Can you work these out from the model? Positions are in its coordinate system, mm. Face numbers are marked on the shaded views. A direction names the side the tool comes from. Give positions to 0.01 mm unless a question says otherwise; leave off trailing zeros. Write each loop counter-clockwise with the first axis right and the second up, starting at its lowest first coordinate (ties: lowest second). Pieces come first, ordered by that corner, then holes.
1. On a 3-axis mill with a long thin cutter (end or side, diameter ignored), from which of +Z, -Z, +X, -X, +Y, -Y can I reach the whole of each face in a straight line? I mean the marked faces 1, 2, 3 and 4. Say none if no direction works.
2. Suppose I cut it at B-B (z = -6.5). Please give me the cut outline in (x, y), and give its area (3 significant figures).
3. Thinking about a two-plate mould opening in X: for the marked faces 5, 6, 7 and 8, which applies, pulls with the +X half, pulls with the -X half, needs draft (parallel to the pull), parting line crosses it, or undercut?
4. I'm going to push flat-ended pins straight in: pin 1 (3 mm diameter, centred on y = -4, z = -6, fed in from -X); pin 2 (3 mm diameter, centred on x = 11, y = -2, fed in from +Z); pin 3 (5 mm diameter, centred on x = 7, z = -4, fed in from +Y); pin 4 (4.5 mm diameter, centred on x = 11, z = 1.5, fed in from -Y). Where does each tip first touch, or does it pass through?
5. Suppose I cut it at D-D (z = 0). Please give me the cut outline in (x, y) (3 decimals), and give its area (3 significant figures).
6. If I drill on probe 1 along X at (y, z) = (1, -6.5); probe 2 along Z at (x, y) = (-10.35, 0.7); probe 3 along X at (y, z) = (8, 0) (3 decimals), over which ranges is the centre line in solid material (lowest first)?
7. Suppose I cut it at C-C (y = -6.5). Please give me the cut outline in (x, z).
8. Suppose I cut it at A-A (x = 10.35). Please give me the cut outline in (y, z).
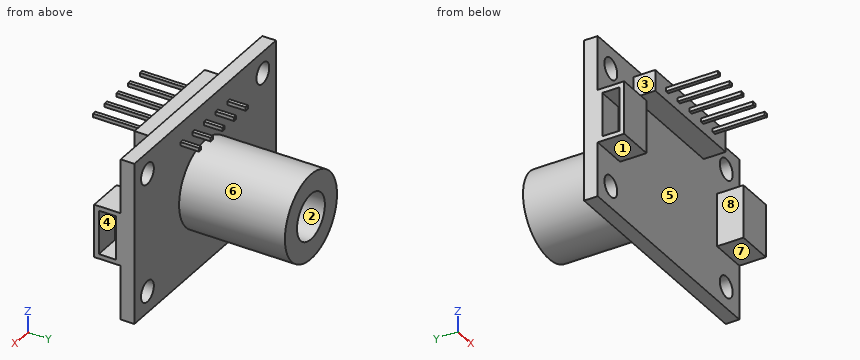
```python
from build123d import *

# Parameters (mm, degrees)
SKETCH1_W                = 25.4
SKETCH1_H                = 17.7
SKETCH1_R                = 1.15
BOSS_EXTRUDE1_DEPTH      = 1.5
SKETCH2_R                = 4.675
BOSS_EXTRUDE2_DEPTH      = 11.6
SKETCH3_R                = 2.5
CUT_EXTRUDE1_DEPTH       = 8
SKETCH4_W                = 4
SKETCH4_H                = 5.8
BOSS_EXTRUDE3_DEPTH      = 2.9
SKETCH5_W                = 4.8
SKETCH5_H                = 1.9
CUT_EXTRUDE2_DEPTH       = 2.9
SKETCH6_W                = 12.6
SKETCH6_H                = 2.3
BOSS_EXTRUDE4_DEPTH      = 2.4
SKETCH7_W                = 0.4
SKETCH7_H                = 0.4
BOSS_EXTRUDE5_DEPTH      = 5.7
BOSS_EXTRUDE5_DEPTH_BACK = 5.9


with BuildPart() as part:
    # Sketch1 → Boss-Extrude1 (new body)
    with BuildSketch(Plane(origin=(0, 0, 0), x_dir=(1, 0, 0), z_dir=(0, 1, 0))):
        Rectangle(SKETCH1_W, SKETCH1_H)
        with Locations((10.35, 6.5)):
            Circle(SKETCH1_R, mode=Mode.SUBTRACT)
        with Locations((10.35, -6.5)):
            Circle(SKETCH1_R, mode=Mode.SUBTRACT)
        with Locations((-10.35, -6.5)):
            Circle(SKETCH1_R, mode=Mode.SUBTRACT)
        with Locations((-10.35, 6.5)):
            Circle(SKETCH1_R, mode=Mode.SUBTRACT)
    extrude(amount=BOSS_EXTRUDE1_DEPTH)

    # Sketch2 → Boss-Extrude2 (add)
    with BuildSketch(Plane(origin=(0, 1.5, 0), x_dir=(1, 0, 0), z_dir=(0, 1, 0))):
        Circle(SKETCH2_R)
    extrude(amount=BOSS_EXTRUDE2_DEPTH)

    # Sketch3 → Cut-Extrude1 (cut)
    with BuildSketch(Plane(origin=(0, 13.1, 0), x_dir=(1, 0, 0), z_dir=(0, 1, 0))):
        Circle(SKETCH3_R)
    extrude(amount=-CUT_EXTRUDE1_DEPTH, mode=Mode.SUBTRACT)

    # Sketch4 → Boss-Extrude3 (add)
    with BuildSketch(Plane.XZ):
        with Locations((10.7, 0)):
            Rectangle(SKETCH4_W, SKETCH4_H)
        with Locations((-10.7, 0)):
            Rectangle(SKETCH4_W, SKETCH4_H)
    extrude(amount=BOSS_EXTRUDE3_DEPTH)

    # Sketch5 → Cut-Extrude2 (cut)
    with BuildSketch(Plane(origin=(12.7, 0, 0), x_dir=(0, 0, -1), z_dir=(1, 0, 0))):
        with Locations((0, -1.45)):
            Rectangle(SKETCH5_W, SKETCH5_H)
    cut_extrude2 = extrude(amount=-CUT_EXTRUDE2_DEPTH, mode=Mode.SUBTRACT)

    # Mirror1: Cut-Extrude2 across plane
    add(cut_extrude2.mirror(Plane(origin=(0, 0, 0), x_dir=(0, 0, 1), z_dir=(1, 0, 0))), mode=Mode.SUBTRACT)

    # Sketch6 → Boss-Extrude4 (add)
    with BuildSketch(Plane.XZ):
        with Locations((0, 6.6)):
            Rectangle(SKETCH6_W, SKETCH6_H)
    extrude(amount=BOSS_EXTRUDE4_DEPTH)

    # Sketch7 → Boss-Extrude5 (add, two sides)
    with BuildSketch(Plane.XZ.offset(2.4)) as boss_extrude5_sk:
        with Locations((-4.2, 6.6)):
            Rectangle(SKETCH7_W, SKETCH7_H)
        with Locations((-2.1, 6.6)):
            Rectangle(SKETCH7_W, SKETCH7_H)
        with Locations((0, 6.6)):
            Rectangle(SKETCH7_W, SKETCH7_H)
        with Locations((2.1, 6.6)):
            Rectangle(SKETCH7_W, SKETCH7_H)
        with Locations((4.2, 6.6)):
            Rectangle(SKETCH7_W, SKETCH7_H)
    extrude(amount=BOSS_EXTRUDE5_DEPTH)
    extrude(boss_extrude5_sk.sketch, amount=-BOSS_EXTRUDE5_DEPTH_BACK)


solid = part.part
```
Checks:
1. face 1: -Z, +X, -X, -Y
1. face 2: +Y
1. face 3: +Z, -Z, -X, -Y
1. face 4: +X
2. outline: (-12.7, 0) - (-11.5, 0) - (-11.5, 1.5) - (-12.7, 1.5) - close; (-9.2, 0) - (9.2, 0) - (9.2, 1.5) - (-9.2, 1.5) - close; (11.5, 0) - (12.7, 0) - (12.7, 1.5) - (11.5, 1.5) - close
2. area: 31.2 mm2
3. face 5: undercut
3. face 6: parting line crosses it
3. face 7: needs draft
3. face 8: undercut
4. pin 1: passes through
4. pin 2: stops at z = 2.9
4. pin 3: stops at y = 1.5
4. pin 4: stops at y = -2.9
5. outline: (-12.7, -2.9) - (-8.7, -2.9) - (-8.7, 0) - (8.7, 0) - (8.7, -2.9) - (12.7, -2.9) - (12.7, -2.4) - (9.8, -2.4) - (9.8, -0.5) - (12.7, -0.5) - (12.7, 1.5) - (4.675, 1.5) - (4.675, 13.1) - (2.5, 13.1) - (2.5, 5.1) - (-2.5, 5.1) - (-2.5, 13.1) - (-4.675, 13.1) - (-4.675, 1.5) - (-12.7, 1.5) - (-12.7, -0.5) - (-9.8, -0.5) - (-9.8, -2.4) - (-12.7, -2.4) - close
5. area: 119 mm2
6. probe 1: x = -12.7 to -11.5, -9.2 to 9.2, 11.5 to 12.7
6. probe 2: z = -8.85 to -7.65, -5.35 to 5.35, 7.65 to 8.85
6. probe 3: x = -4.675 to -2.5, 2.5 to 4.675
7. outline: (-4.4, 6.4) - (-4, 6.4) - (-4, 6.8) - (-4.4, 6.8) - close; (-2.3, 6.4) - (-1.9, 6.4) - (-1.9, 6.8) - (-2.3, 6.8) - close; (-0.2, 6.4) - (0.2, 6.4) - (0.2, 6.8) - (-0.2, 6.8) - close; (1.9, 6.4) - (2.3, 6.4) - (2.3, 6.8) - (1.9, 6.8) - close; (4, 6.4) - (4.4, 6.4) - (4.4, 6.8) - (4, 6.8) - close
8. outline: (-2.9, -2.9) - (0, -2.9) - (0, -5.35) - (1.5, -5.35) - (1.5, 5.35) - (0, 5.35) - (0, 2.9) - (-2.9, 2.9) - close; (0, -8.85) - (1.5, -8.85) - (1.5, -7.65) - (0, -7.65) - close; (0, 7.65) - (1.5, 7.65) - (1.5, 8.85) - (0, 8.85) - close; hole (-2.4, -2.4) - (-0.5, -2.4) - (-0.5, 2.4) - (-2.4, 2.4) - close
